Geometry check sheet. Reference: the model listing, model coordinates, mm. A direction names the side the tool comes from. Round coordinates to 2 decimals unless told otherwise and drop trailing zeros. Write each loop counter-clockwise with the first axis right and the second up, starting at its lowest first coordinate (ties: lowest second). Pieces come first, ordered by that corner, then holes. Notation, with made-up numbers: (9, 87.25) - (19, 87.25) arc R6 cw to (19, 98.25) - close; hole circle Ø10 at (20, 37). An arc over 180 degrees is marked (long way). Return JSON: item names as keys, results as strings.
```python
from build123d import *

# Parameters (mm, degrees)
SKETCH_1_R               = 5
EXTRUDE_1_DEPTH          = 130
EXTRUDE_START            = -35
SKETCH_2_R               = 10
EXTRUDE_2_DEPTH          = 60
CUT_EXTRUDE_1_DEPTH      = 131.766968306
CUT_EXTRUDE_1_DEPTH_BACK = 131.766968306
SKETCH_3_R               = 1.6


with BuildPart() as part:
    # 草图1 → 凸台-拉伸1 (new body)
    with BuildSketch(Plane.XY):
        Circle(SKETCH_1_R)
    extrude(amount=EXTRUDE_1_DEPTH)

    # 草图2 → 凸台-拉伸2 (add)
    with BuildSketch(Plane.XY.offset(130).offset(EXTRUDE_START)):
        Circle(SKETCH_2_R)
    extrude(amount=-EXTRUDE_2_DEPTH)

    # 草图3 → 切除-拉伸1 (cut, two sides: drawn at the far end of the back side and taken through both)
    with BuildSketch(Plane(origin=(0, 0, 0), x_dir=(1, 0, 0), z_dir=(0, 1, 0)).offset(-CUT_EXTRUDE_1_DEPTH_BACK)):
        with Locations(Location((0, -125, 0), (0, 0, 270))):
            Circle(SKETCH_3_R)
        with Locations(Location((0, -5, 0), (0, 0, 270))):
            Circle(SKETCH_3_R)
    extrude(amount=CUT_EXTRUDE_1_DEPTH + CUT_EXTRUDE_1_DEPTH_BACK, mode=Mode.SUBTRACT)


solid = part.part
```
(1) Gauge pin test, flat ends, axial feed: pin 1 (1.5 mm diameter, centred on x = -7.5, y = -0.5, fed in from +Z); pin 2 (12 mm diameter, centred on x = 7.5, z = 68, fed in from -Y); pin 3 (1.5 mm diameter, centred on x = 5, z = 90.5, fed in from +Y); pin 4 (2.5 mm diameter, centred on x = 0, z = 125, fed in from +Y). Record the tip position at first contact, or that the pin passes through.
Response values:
{"pin 1": "stops at z = 95", "pin 2": "stops at y = -9.89", "pin 3": "stops at y = 9.05", "pin 4": "passes through"}
(2) Release check for a two-part mould opening along Z. For faces 4 (the face through (-0.61, -0.07, 6.48)), 5 (the face through (-5, -2, 35)), 6 (the face through (0, 0, 130)) record: pulls with the +Z half, pulls with the -Z half, needs draft (parallel to the pull), parting line crosses it, or undercut.
Response values:
{"face 4": "undercut", "face 5": "pulls with the -Z half", "face 6": "pulls with the +Z half"}
(3) Section check B-B, the plane y = 0. Enter the section's corners in (x, z).
Response values:
{"outline": "(-10, 35) - (-5, 35) - (-5, 0) - (5, 0) - (5, 35) - (10, 35) - (10, 95) - (5, 95) - (5, 130) - (-5, 130) - (-5, 95) - (-10, 95) - close; hole circle Ø3.2 at (0, 5); hole circle Ø3.2 at (0, 125)"}
(4) Section check A-A, the plane x = 0. Enter the section's corners in (y, z), plus the area to 3 significant figures.
Response values:
{"outline": "(-10, 35) - (-5, 35) - (-5, 6.6) - (5, 6.6) - (5, 35) - (10, 35) - (10, 95) - (5, 95) - (5, 123.4) - (-5, 123.4) - (-5, 95) - (-10, 95) - close; (-5, 0) - (5, 0) - (5, 3.4) - (-5, 3.4) - close; (-5, 126.6) - (5, 126.6) - (5, 130) - (-5, 130) - close", "area": "1,840 mm^2"}
(5) Section check D-D, the plane z = 125. Enter the section's corners in (x, y).
Response values:
{"outline": "(-1.6, -4.74) - (-1.6, 4.74) arc R5 ccw to start; (1.6, -4.74) arc R5 ccw to (1.6, 4.74) - close"}
(6) Section check C-C, the plane z = 20. Enter the section's corners in (x, y).
Response values:
{"outline": "circle Ø10 at (0, 0)"}
(7) Material ranges on line 1 along Z through (x, y) = (0, 2.25); line 2 along X through (y, z) = (0, 5); line 3 along Z through (x, y) = (-8.25, 4.25), recorded low to high. Write a range as [from, to].
Response values:
{"line 1": "z = [0, 3.4], [6.6, 123.4], [126.6, 130]", "line 2": "x = [-5, -1.6], [1.6, 5]", "line 3": "z = [35, 95]"}
(8) Access from +Z, -Z, +X, -X, +Y, -Y to the whole of each face (thin tool, end or side, straight path). Record for faces 1 (the face through (4.77, 1.5, 112.26)), 2 (the face through (4.77, 1.5, 17.26)), 3 (the face through (0, 0, 0)).
Response values:
{"face 1": "+Z", "face 2": "-Z", "face 3": "-Z, +X, -X, +Y, -Y"}
